Verification items for this drawing (mm, ordinates from the low corner). A direction names the side the tool comes from. Give positions to 0.01 mm unless a question says otherwise; leave off trailing zeros. Loops run counter-clockwise (first coordinate to the right, second up) from the corner with the lowest first, then second, coordinate; pieces in that order, holes last. Notation, with made-up numbers: (28, -14) -> (41, -14) arc R23 ccw to (41, 2) -> close; hole circle Ø8 at (-23.5, -7). An arc over 180 degrees is marked (long way). Write item = value, one per line.
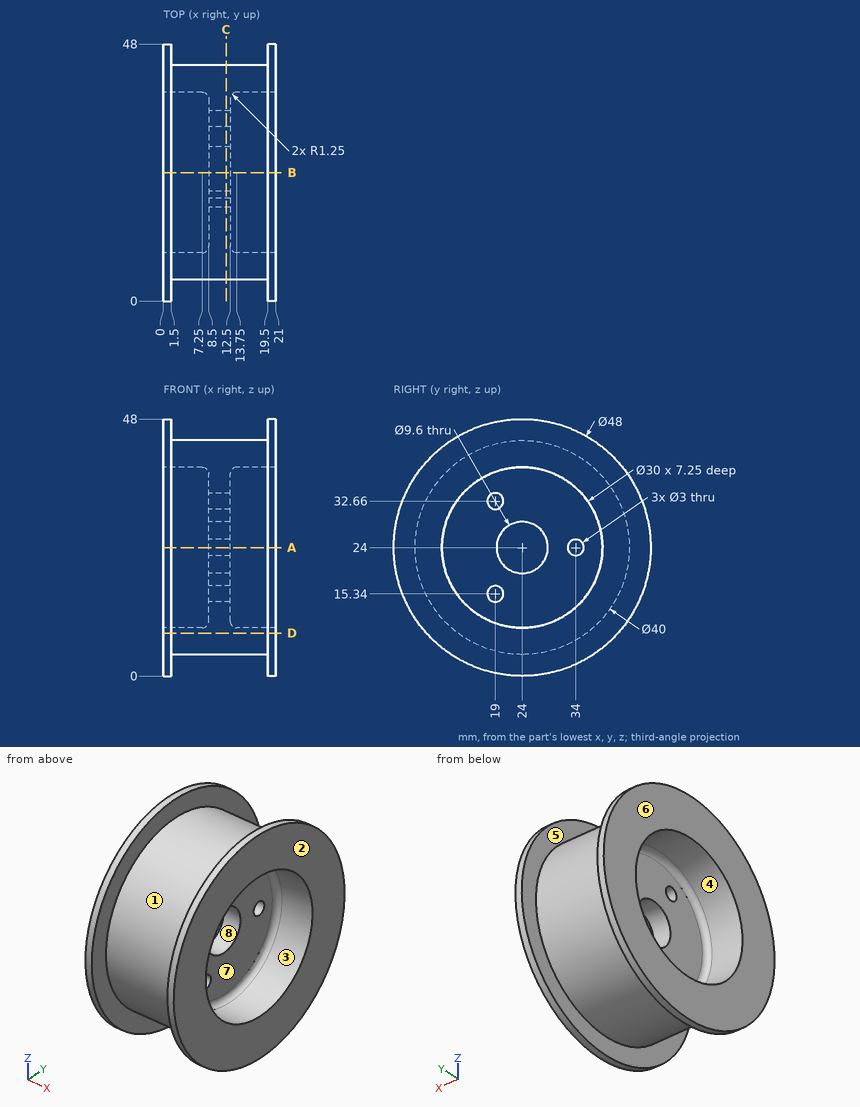
Item 1: Section check C-C, the plane x = 11.75. Record the cut outline in (y, z), plus the area to 3 significant figures.
Answer:
outline = circle Ø40 at (24, 24); hole circle Ø3 at (19, 15.34); hole circle Ø3 at (19, 32.66); hole circle Ø9.6 at (24, 24); hole circle Ø3 at (34, 24)
area = 1,160 mm^2
Item 2: Thickness scan on L1, parallel to Y at x = 9.85, z = 24; L2, parallel to Y at x = 5.25, z = 24; L3, parallel to Y at x = 19.75, z = 34.5. Record the ranges inside material, lowest first. Write a range as [from, to].
Answer:
L1 = [4, 19.2], [28.8, 32.5], [35.5, 44]
L2 = [4, 9], [39, 44]
L3 = [2.42, 13.29], [34.71, 45.58]
Item 3: Section check A-A, the plane z = 24. Give the number of separate pieces and of enclosed holes in the cut face, plus the area to 3 significant figures.
Answer:
separate_pieces = 3
enclosed_holes = 0
area = 305 mm^2
Item 4: Section check B-B, the plane y = 24. Record the cut outline in (x, z).
Answer:
outline = (0, 0) -> (1.5, 0) -> (1.5, 4) -> (19.5, 4) -> (19.5, 0) -> (21, 0) -> (21, 9) -> (13.75, 9) arc R1.25 cw to (12.5, 10.25) -> (12.5, 19.2) -> (8.5, 19.2) -> (8.5, 10.25) arc R1.25 cw to (7.25, 9) -> (0, 9) -> close; (0, 39) -> (7.25, 39) arc R1.25 cw to (8.5, 37.75) -> (8.5, 28.8) -> (12.5, 28.8) -> (12.5, 37.75) arc R1.25 cw to (13.75, 39) -> (21, 39) -> (21, 48) -> (19.5, 48) -> (19.5, 44) -> (1.5, 44) -> (1.5, 48) -> (0, 48) -> close
Item 5: Draft check along Y on the marked faces 1, 2 and 3. Enter one of: +Y half, -Y half, draft (parallel to the pull), parting line (faces both ways), or undercut.
Answer:
face_1 = parting line
face_2 = draft
face_3 = undercut
Item 6: Tool access check on the marked faces 4, 5, 6, 7 and 8. Record the directions out of +Z, -Z, +X, -X, +Y, -Y that give a thin tool (end or side, any length) a straight path to the whole face; none if there is none.
Answer:
face_4 = -X
face_5 = none
face_6 = +Z, -Z, -X, +Y, -Y
face_7 = +X
face_8 = +X, -X
Item 7: Section check D-D, the plane z = 8. Record the cut outline in (x, y).
Answer:
outline = (0, 6.11) -> (1.5, 6.11) -> (1.5, 12) -> (19.5, 12) -> (19.5, 6.11) -> (21, 6.11) -> (21, 41.89) -> (19.5, 41.89) -> (19.5, 36) -> (1.5, 36) -> (1.5, 41.89) -> (0, 41.89) -> close
Item 8: Gauge pin test, flat ends, axial feed: pin 1 (6 mm diameter, centred on x = 17.5, y = 35.5, fed in from -Z); pin 2 (8 mm diameter, centred on y = 29, z = 21, fed in from +X); pin 3 (14 mm diameter, centred on y = 18, z = 19.5, fed in from -X). Record the tip position at first contact, or that the pin passes through.
Answer:
pin_1 = 1.86
pin_2 = 12.5
pin_3 = 8.25
